Input: part model. Units: mm. Frame: model coordinates. A direction names the side the tool comes from. Coordinates: 2 decimals unless noted, no trailing zeros. Order: outer loops, then holes, each group sorted by start corner. A loop starts at its lowest first (then second) coordinate and runs counter-clockwise, first axis right, second up. Notation, with made-up numbers: (-29.75, 48.25) - (-13.75, 48.25) arc R10 ccw to (-13.75, 61.25) - close; hole circle Ø2 at (-34.5, 85.5). An arc over 180 degrees is marked (long way). Answer as CSV lines item,"result". Start each with the question number.
Item 1: First-contact query: pin 1 (8 mm diameter, centred on x = 9, z = 16, fed in from +Y); pin 2 (1.5 mm diameter, centred on x = -0.5, z = 52, fed in from +Y); pin 3 (0.5 mm diameter, centred on x = -2, y = 3.5, fed in from -Z). Flat tips, straight axial feed; report the tip coordinate or a pass-through.
Item 2: Section A-A (x = 16.5). Output: boundary loops of the cut face in (y, z).
Item 3: Material intervals for line 1 along Z through (x, y) = (0, 2.85); line 2 along Y through (x, z) = (-3, 31.5); line 3 along Y through (x, z) = (3.5, -64), sorted ascending.
Item 4: Section B-B (z = 26). Output: boundary loops of the cut face in (x, y).
Item 5: Access query for faces 5 (the flat face through (0, -2.5, 1)), 6 (the flat face through (-1, 2.7, 52)), 7 (the flat face through (0, 0, -56)). Directions: +Z, -Z, +X, -X, +Y, -Y. A direction counts if a zero-diameter tool reaches every point of the face in a straight line with its end or side. Return the directions, or none.
Item 6: Draft query along Y for faces 1 (the flat face through (-4, 0, -64)), 2 (the flat face through (4, 0, -64)), 3 (the flat face through (1, 0, 72)), 4 (the flat face through (0, 4, 55)). Return one class per face: +Y half, -Y half, draft (parallel to the pull), parting line (faces both ways), or undercut.
from build123d import *

# Parameters (mm, degrees)
F0_W      = 72.5
F0_H      = 144
F1_DEPTH  = 3
F2_W      = 72.5
F2_H      = 144
F3_DEPTH  = 3
F5_W      = 15
F5_H      = 5
F6_DEPTH  = 0.3
F7_W      = 8
F7_H      = 4
F8_DEPTH  = 16
F9_W      = 13
F9_H      = 1
F10_DEPTH = 1
F11_W     = 11
F11_H     = 11
F12_DEPTH = 1
F13_R     = 2.5
F14_DEPTH = 1
F4_W      = 66
F4_H      = 116.5
F15_DEPTH = 0.5
F16_R     = 1.481304
F17_DEPTH = 0.3
F18_R     = 0.686306
F19_DEPTH = 0.1


with BuildPart() as f1:
    # F0 (on Front) → F1 (new body)
    with BuildSketch(Plane.XZ):
        Rectangle(F0_W, F0_H)
    extrude(amount=F1_DEPTH)

    # F2 (on face) → F3 (join)
    with BuildSketch(Plane(origin=(0, 0, 0), x_dir=(-1, 0, 0), z_dir=(0, 1, 0))):
        Rectangle(F2_W, F2_H)
    extrude(amount=F3_DEPTH)

    # F5 (on face) → F6 (join)
    with BuildSketch(Plane.XZ.offset(3)):
        with Locations((0, -65.126628)):
            Rectangle(F5_W, F5_H)
    extrude(amount=F6_DEPTH)

    # F7 (on face) → F8 (cut)
    with BuildSketch(Plane(origin=(0, 0, -72), x_dir=(1, 0, 0), z_dir=(0, 0, -1))):
        Rectangle(F7_W, F7_H)
    extrude(amount=-F8_DEPTH, mode=Mode.SUBTRACT)

    # F9 (on face) → F10 (cut)
    with BuildSketch(Plane.XZ.offset(3)):
        with Locations((0, 68.084061)):
            Rectangle(F9_W, F9_H)
    extrude(amount=-F10_DEPTH, mode=Mode.SUBTRACT)

    # F11 (on face) → F12 (join)
    with BuildSketch(Plane(origin=(0, 3, 0), x_dir=(-1, 0, 0), z_dir=(0, 1, 0))):
        with Locations((0, 52.234016)):
            Rectangle(F11_W, F11_H)
    extrude(amount=F12_DEPTH)

    # F13 (on face) → F14 (cut)
    with BuildSketch(Plane(origin=(0, 4, 0), x_dir=(-1, 0, 0), z_dir=(0, 1, 0))):
        with Locations((0, 52.198544)):
            Circle(F13_R)
    extrude(amount=-F14_DEPTH, mode=Mode.SUBTRACT)

    # F4 (on face) → F15 (cut)
    with BuildSketch(Plane.XZ.offset(3)):
        Rectangle(F4_W, F4_H)
    extrude(amount=-F15_DEPTH, mode=Mode.SUBTRACT)

    # F16 (on face) → F17 (cut)
    with BuildSketch(Plane(origin=(0, 3, 0), x_dir=(-1, 0, 0), z_dir=(0, 1, 0))):
        with Locations((0, 52.198544)):
            Circle(F16_R)
    extrude(amount=-F17_DEPTH, mode=Mode.SUBTRACT)

    # F18 (on face) → F19 (join)
    with BuildSketch(Plane(origin=(0, 2.7, 0), x_dir=(-1, 0, 0), z_dir=(0, 1, 0))):
        with Locations((0, 52.198544)):
            Circle(F18_R)
    extrude(amount=F19_DEPTH)


solid = f1.part
Determined:
1,pin 1,"stops at y = 3"
1,pin 2,"stops at y = 2.8"
1,pin 3,"stops at z = 46.73"
2,outline,"(-3, -72) - (3, -72) - (3, 72) - (-3, 72) - (-3, 58.25) - (-2.5, 58.25) - (-2.5, -58.25) - (-3, -58.25) - close"
3,line 1,"z = -72 to 50.72, 53.68 to 72"
3,line 2,"y = -2.5 to 3"
3,line 3,"y = -3.3 to -2, 2 to 3"
4,outline,"(-36.25, -3) - (-33, -3) - (-33, -2.5) - (33, -2.5) - (33, -3) - (36.25, -3) - (36.25, 3) - (-36.25, 3) - close"
5,face 5,"-Y"
5,face 6,"+Y"
5,face 7,"-Z"
6,face 1,"undercut"
6,face 2,"undercut"
6,face 3,"draft"
6,face 4,"+Y half"
